```python
from build123d import *

# Parameters (mm, degrees)
SKETCH1_R           = 90
SKETCH1_R_2         = 71.5
BOSS_EXTRUDE1_DEPTH = 5
SKETCH1_4_R         = 1.55
CUT_EXTRUDE1_DEPTH  = 5
SKETCH1_5_R         = 3.5
SKETCH1_5_R_2       = 1.55
CUT_EXTRUDE2_DEPTH  = 2.5
FILLET1_R           = 5


with BuildPart() as part:
    # Sketch1 → Boss-Extrude1 (new body)
    with BuildSketch(Plane(origin=(0, 0, 0), x_dir=(1, 0, 0), z_dir=(0, 1, 0))):
        with Locations(Location((0, 0, 0), (0, 0, 270))):
            Circle(SKETCH1_R)
        with Locations(Location((0, 0, 0), (0, 0, 270))):
            Circle(SKETCH1_R_2, mode=Mode.SUBTRACT)
    extrude(amount=-BOSS_EXTRUDE1_DEPTH)

    # Sketch1<4> → Cut-Extrude1 (cut)
    with BuildSketch(Plane(origin=(0, 0, 0), x_dir=(1, 0, 0), z_dir=(0, 1, 0))):
        with Locations(Location((0, -85.5, 0), (0, 0, 270))):
            Circle(SKETCH1_4_R)
        with Locations(Location((-74.045172024, -42.75, 0), (0, 0, 270))):
            Circle(SKETCH1_4_R)
        with Locations(Location((-42.75, -74.045172024, 0), (0, 0, 270))):
            Circle(SKETCH1_4_R)
        with Locations(Location((-85.5, 0, 0), (0, 0, 270))):
            Circle(SKETCH1_4_R)
        with Locations(Location((-74.045172024, 42.75, 0), (0, 0, 270))):
            Circle(SKETCH1_4_R)
        with Locations(Location((-42.75, 74.045172024, 0), (0, 0, 270))):
            Circle(SKETCH1_4_R)
        with Locations(Location((0, 85.5, 0), (0, 0, 270))):
            Circle(SKETCH1_4_R)
        with Locations(Location((42.75, 74.045172024, 0), (0, 0, 270))):
            Circle(SKETCH1_4_R)
        with Locations(Location((74.045172024, 42.75, 0), (0, 0, 270))):
            Circle(SKETCH1_4_R)
        with Locations(Location((85.5, 0, 0), (0, 0, 270))):
            Circle(SKETCH1_4_R)
        with Locations(Location((74.045172024, -42.75, 0), (0, 0, 270))):
            Circle(SKETCH1_4_R)
        with Locations(Location((42.75, -74.045172024, 0), (0, 0, 270))):
            Circle(SKETCH1_4_R)
    extrude(amount=-CUT_EXTRUDE1_DEPTH, mode=Mode.SUBTRACT)

    # Sketch1<5> → Cut-Extrude2 (cut)
    # profile 1 of 12: a face of its own
    with BuildSketch(Plane(origin=(0, 0, 0), x_dir=(1, 0, 0), z_dir=(0, 1, 0))):
        with Locations(Location((-74.045172024, -42.75, 0), (0, 0, 270))):
            Circle(SKETCH1_5_R)
        with Locations(Location((-74.045172024, -42.75, 0), (0, 0, 270))):
            Circle(SKETCH1_5_R_2, mode=Mode.SUBTRACT)
    # profile 2 of 12: a face of its own
    with BuildSketch(Plane(origin=(0, 0, 0), x_dir=(1, 0, 0), z_dir=(0, 1, 0))):
        with Locations(Location((-85.5, 0, 0), (0, 0, 270))):
            Circle(SKETCH1_5_R)
        with Locations(Location((-85.5, 0, 0), (0, 0, 270))):
            Circle(SKETCH1_5_R_2, mode=Mode.SUBTRACT)
    # profile 3 of 12: a face of its own
    with BuildSketch(Plane(origin=(0, 0, 0), x_dir=(1, 0, 0), z_dir=(0, 1, 0))):
        with Locations(Location((-42.75, -74.045172024, 0), (0, 0, 270))):
            Circle(SKETCH1_5_R)
        with Locations(Location((-42.75, -74.045172024, 0), (0, 0, 270))):
            Circle(SKETCH1_5_R_2, mode=Mode.SUBTRACT)
    # profile 4 of 12: a face of its own
    with BuildSketch(Plane(origin=(0, 0, 0), x_dir=(1, 0, 0), z_dir=(0, 1, 0))):
        with Locations(Location((0, -85.5, 0), (0, 0, 270))):
            Circle(SKETCH1_5_R)
        with Locations(Location((0, -85.5, 0), (0, 0, 270))):
            Circle(SKETCH1_5_R_2, mode=Mode.SUBTRACT)
    # profile 5 of 12: a face of its own
    with BuildSketch(Plane(origin=(0, 0, 0), x_dir=(1, 0, 0), z_dir=(0, 1, 0))):
        with Locations(Location((-74.045172024, 42.75, 0), (0, 0, 270))):
            Circle(SKETCH1_5_R)
        with Locations(Location((-74.045172024, 42.75, 0), (0, 0, 270))):
            Circle(SKETCH1_5_R_2, mode=Mode.SUBTRACT)
    # profile 6 of 12: a face of its own
    with BuildSketch(Plane(origin=(0, 0, 0), x_dir=(1, 0, 0), z_dir=(0, 1, 0))):
        with Locations(Location((-42.75, 74.045172024, 0), (0, 0, 270))):
            Circle(SKETCH1_5_R)
        with Locations(Location((-42.75, 74.045172024, 0), (0, 0, 270))):
            Circle(SKETCH1_5_R_2, mode=Mode.SUBTRACT)
    # profile 7 of 12: a face of its own
    with BuildSketch(Plane(origin=(0, 0, 0), x_dir=(1, 0, 0), z_dir=(0, 1, 0))):
        with Locations(Location((0, 85.5, 0), (0, 0, 270))):
            Circle(SKETCH1_5_R)
        with Locations(Location((0, 85.5, 0), (0, 0, 270))):
            Circle(SKETCH1_5_R_2, mode=Mode.SUBTRACT)
    # profile 8 of 12: a face of its own
    with BuildSketch(Plane(origin=(0, 0, 0), x_dir=(1, 0, 0), z_dir=(0, 1, 0))):
        with Locations(Location((74.045172024, 42.75, 0), (0, 0, 270))):
            Circle(SKETCH1_5_R)
        with Locations(Location((74.045172024, 42.75, 0), (0, 0, 270))):
            Circle(SKETCH1_5_R_2, mode=Mode.SUBTRACT)
    # profile 9 of 12: a face of its own
    with BuildSketch(Plane(origin=(0, 0, 0), x_dir=(1, 0, 0), z_dir=(0, 1, 0))):
        with Locations(Location((42.75, 74.045172024, 0), (0, 0, 270))):
            Circle(SKETCH1_5_R)
        with Locations(Location((42.75, 74.045172024, 0), (0, 0, 270))):
            Circle(SKETCH1_5_R_2, mode=Mode.SUBTRACT)
    # profile 10 of 12: a face of its own
    with BuildSketch(Plane(origin=(0, 0, 0), x_dir=(1, 0, 0), z_dir=(0, 1, 0))):
        with Locations(Location((74.045172024, -42.75, 0), (0, 0, 270))):
            Circle(SKETCH1_5_R)
        with Locations(Location((74.045172024, -42.75, 0), (0, 0, 270))):
            Circle(SKETCH1_5_R_2, mode=Mode.SUBTRACT)
    # profile 11 of 12: a face of its own
    with BuildSketch(Plane(origin=(0, 0, 0), x_dir=(1, 0, 0), z_dir=(0, 1, 0))):
        with Locations(Location((85.5, 0, 0), (0, 0, 270))):
            Circle(SKETCH1_5_R)
        with Locations(Location((85.5, 0, 0), (0, 0, 270))):
            Circle(SKETCH1_5_R_2, mode=Mode.SUBTRACT)
    # profile 12 of 12: a face of its own
    with BuildSketch(Plane(origin=(0, 0, 0), x_dir=(1, 0, 0), z_dir=(0, 1, 0))):
        with Locations(Location((42.75, -74.045172024, 0), (0, 0, 270))):
            Circle(SKETCH1_5_R)
        with Locations(Location((42.75, -74.045172024, 0), (0, 0, 270))):
            Circle(SKETCH1_5_R_2, mode=Mode.SUBTRACT)
    extrude(amount=-CUT_EXTRUDE2_DEPTH, mode=Mode.SUBTRACT)

    # Sketch2 → Revolve1 (revolve)
    with BuildSketch(Plane.XY, mode=Mode.PRIVATE) as revolve1_sk:
        with BuildLine():
            Line((0, 65), (0, 62))
            ThreePointArc((0, 62), (47.507894081, 44.364006029), (72, 0))
            Line((72, 0), (75, 0))
            ThreePointArc((75, 0), (49.623583103, 46.488749734), (0, 65))
        make_face()
    revolve(revolve1_sk.sketch.rotate(Axis((0, 0, 0), (0, 1, 0)), 180), axis=Axis((0, 0, 0), (0, 1, 0)))

    # Fillet1
    fillet1_edges = [part.edges().sort_by_distance(p)[0] for p in [
        (75, 0, 0),
        (0, -5, -71.5),
    ]]
    fillet(fillet1_edges, radius=FILLET1_R - 0.0001)  # a hair under: the kernel refuses the full size


solid = part.part
```
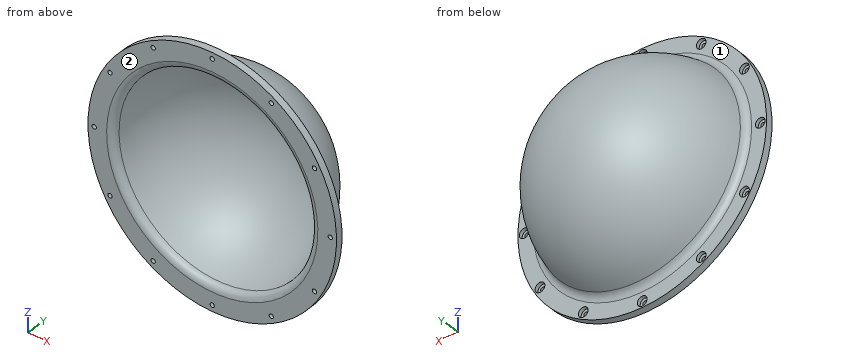
Work out the finished part from the listing and answer in its coordinate system (mm). Face numbers are marked on the shaded views. A direction names the side the tool comes from. Coordinates: 2 decimals unless noted, no trailing zeros. Order: outer loops, then holes, each group sorted by start corner. A loop starts at its lowest first (then second) coordinate and runs counter-clockwise, first axis right, second up. Notation, with made-up numbers: M -26,-12 L 27,-12 A20 cw 27,-5 Z; hole C 61,71.5 d10. An arc over 180 degrees is marked long. Use CSV: the item, a comma, the result in double quotes.
1) Flat-ended cylindrical pins translate along their axes: pin 1 Ø5.5 at (x, z) = (-74.05, -42.75) entering from +Y; pin 2 Ø1 at (x, z) = (60, -24.5) entering from +Y; pin 3 Ø1 at (y, z) = (28, -13.5) entering from -X. Find the tip coordinate at first contact, or state that the pin passes through.
Worked out:
pin 1,"stops at y = -2.5"
pin 2,"stops at y = 29.3"
pin 3,"stops at x = -64"
2) Consider line 1 (X direction, y = -1, z = -42.75); line 2 (X direction, y = -3.1, z = 42.75); line 3 (Z direction, x = 25.5, y = 29). Determine where each line is inside the solid, lowest interval first. Write a range as [from, to].
Worked out:
line 1,"x = [-79.2, -77.55], [-70.55, -57.44], [57.44, 70.55], [77.55, 79.2]"
line 2,"x = [-79.2, -75.6], [-72.5, -58.65], [58.65, 72.5], [75.6, 79.2]"
line 3,"z = [-59.24, -55.37], [55.37, 59.24]"
3) Section B-B on y = 45.5 is taken. Write down the section's boundary in (x, z), plus the area to 3 significant figures.
Worked out:
outline,"C 0,0 d101.48; hole C 0,0 d92.31"
area,"1,400 mm^2"
4) Section A-A on y = 32.5 is taken. Write down the section's boundary in (x, z), plus the area to 3 significant figures.
Worked out:
outline,"C 0,0 d124.4; hole C 0,0 d117.05"
area,"1,390 mm^2"
5) For the marked faces 1 and 2, determine the directions among +Z, -Z, +X, -X, +Y, -Y from which every point of the face is accessible in a straight line to the end or side of a thin tool.
Worked out:
face 1,"+Y"
face 2,"+Z, -Z, +X, -X, -Y"
